```python
from build123d import *

# Parameters (mm, degrees)
SKETCH1_R           = 2.25
SKETCH1_R_2         = 8
SKETCH1_R_3         = 2.5
BOSS_EXTRUDE1_DEPTH = 1.5


with BuildPart() as part:
    # Sketch1 → Boss-Extrude1 (new body)
    with BuildSketch(Plane.XY):
        with BuildLine():
            Line((15, 13.228756555), (17.79, 13.228756555))
            Line((17.79, 13.228756555), (37.79, 13.228756555))
            Line((37.79, 13.228756555), (37.79, -13.228756555))
            Line((37.79, -13.228756555), (17.79, -13.228756555))
            Line((17.79, -13.228756555), (15, -13.228756555))
            ThreePointArc((15, -13.228756555), (0, -20), (-15, -13.228756555))
            Line((-15, -13.228756555), (-15, 13.228756555))
            ThreePointArc((-15, 13.228756555), (0, 20), (15, 13.228756555))
        make_face()
        with Locations((-11.313708499, 11.313708499)):
            Circle(SKETCH1_R, mode=Mode.SUBTRACT)
        with Locations((0, 16)):
            Circle(SKETCH1_R, mode=Mode.SUBTRACT)
        with Locations((11.313708499, 11.313708499)):
            Circle(SKETCH1_R, mode=Mode.SUBTRACT)
        with Locations((-11.313708499, -11.313708499)):
            Circle(SKETCH1_R, mode=Mode.SUBTRACT)
        with Locations((0, -16)):
            Circle(SKETCH1_R, mode=Mode.SUBTRACT)
        Circle(SKETCH1_R_2, mode=Mode.SUBTRACT)
        with Locations((11.313708499, -11.313708499)):
            Circle(SKETCH1_R, mode=Mode.SUBTRACT)
        with Locations((27.79, 0)):
            Circle(SKETCH1_R_3, mode=Mode.SUBTRACT)
        with Locations((27.79, 8)):
            Circle(SKETCH1_R_3, mode=Mode.SUBTRACT)
        with Locations((27.79, -8)):
            Circle(SKETCH1_R_3, mode=Mode.SUBTRACT)
    extrude(amount=BOSS_EXTRUDE1_DEPTH)


solid = part.part
```
Geometry check sheet. Reference: the model listing, model coordinates, mm. A direction names the side the tool comes from. Round coordinates to 2 decimals unless told otherwise and drop trailing zeros. Loops run counter-clockwise (first coordinate to the right, second up) from the corner with the lowest first, then second, coordinate; pieces in that order, holes last. Notation, with made-up numbers: (-25.5, 57) - (-5.5, 57) arc R19 ccw to (-5.5, 87) - close; hole circle Ø2 at (89, -26.5). An arc over 180 degrees is marked (long way). Write each question's results on one line, items separated by ' | '. Start each with the question number.
Q1. Cross-section at D-D on z = 0.6. State how many separate pieces and enclosed holes the cut face has, and give its area (3 significant figures).
Q2. Gauge pin test, flat ends, axial feed: P1, Ø2.5, axis at x = -11.31, y = 11.31, coming from the -Z side; P2, Ø0.8, axis at x = 21.5, z = 1, coming from the +Y side. Record the tip position at first contact, or that the pin passes through.
Q3. Thickness scan on line 1 (Y direction, x = 28, z = 1); line 2 (X direction, y = -6, z = 0.35); line 3 (X direction, y = -11, z = 0.7). Record the ranges inside material, lowest first. Write a range as [from, to].
Q4. Cross-section at A-A on x = 27.79. Enter the section's corners in (y, z).
Q5. Cross-section at B-B on y = -16. Enter the section's corners in (x, z), and give its area (4 significant figures).
Q6. Release check for a two-part mould opening along X. For faces 3 (the flat face through (26, 13.229, 1)), 4 (the flat face through (-15, 0, 1)), 5 (the cylindrical face through (12.35, -13.31, 0.74)) record: +X half, -X half, draft (parallel to the pull), parting line (faces both ways), or undercut.
Q7. Cross-section at C-C on y = -1. Enter the section's corners in (x, z), and give its area (3 significant figures).
Q8. Access from +Z, -Z, +X, -X, +Y, -Y to the whole of each face (thin tool, end or side, straight path). Record for faces 1 (the cylindrical face through (-10.1, 13.21, 0.74)), 2 (the flat face through (27, -13.229, 1)).
Answers below:
1) separate pieces: 1 | enclosed holes: 10 | area: 1,320 mm²
2) P1: passes through | P2: stops at y = 13.23
3) line 1: y = [-13.23, -10.49], [-5.51, -2.49], [2.49, 5.51], [10.49, 13.23] | line 2: x = [-15, -5.29], [5.29, 26.29], [29.29, 37.79] | line 3: x = [-15, -13.54], [-9.09, 9.09], [13.54, 37.79]
4) outline: (-13.23, 0) - (-10.5, 0) - (-10.5, 1.5) - (-13.23, 1.5) - close; (-5.5, 0) - (-2.5, 0) - (-2.5, 1.5) - (-5.5, 1.5) - close; (2.5, 0) - (5.5, 0) - (5.5, 1.5) - (2.5, 1.5) - close; (10.5, 0) - (13.23, 0) - (13.23, 1.5) - (10.5, 1.5) - close
5) outline: (-12, 0) - (-2.25, 0) - (-2.25, 1.5) - (-12, 1.5) - close; (2.25, 0) - (12, 0) - (12, 1.5) - (2.25, 1.5) - close | area: 29.25 mm²
6) face 3: draft | face 4: -X half | face 5: undercut
7) outline: (-15, 0) - (-7.94, 0) - (-7.94, 1.5) - (-15, 1.5) - close; (7.94, 0) - (25.5, 0) - (25.5, 1.5) - (7.94, 1.5) - close; (30.08, 0) - (37.79, 0) - (37.79, 1.5) - (30.08, 1.5) - close | area: 48.5 mm²
8) face 1: +Z, -Z | face 2: +Z, -Z, +X, -Y
